Check sheet for the modelled part. Datum: model origin and axes. Units: mm. Face numbers are marked on the shaded views. A direction names the side the tool comes from. Give positions to 0.01 mm unless a question says otherwise; leave off trailing zeros. Order: outer loops, then holes, each group sorted by start corner. A loop starts at its lowest first (then second) coordinate and runs counter-clockwise, first axis right, second up. Notation, with made-up numbers: (-7.5, -0.75) -> (7.5, -0.75) arc R5 ccw to (7.5, 6.25) -> close; hole circle Ø9 at (44, 86.5). An arc over 180 degrees is marked (long way). Answer in a Markdown table with one row per item. Add a question column.
(1) Cross-section at B-B (y = 37). Record the cut outline in (x, z), then the cut area to 3 significant figures.
(2) Release check for a two-part mould opening along X. For the marked faces 3, 4, 5 and 6 record: released by +X, released by -X, zero draft, split by the parting line, or undercut.
(3) Cross-section at D-D (z = 7). Record the cut outline in (x, y), then the cut area to 3 significant figures.
(4) Cross-section at C-C (x = 0). Record the cut outline in (y, z).
(5) Cross-section at A-A (x = 7). Record the cut outline in (y, z).
(6) Set-up check for the marked faces 1 and 2: record each of +Z, -Z, +X, -X, +Y, -Y from which the full face is reachable in a straight line by a thin tool's end or side.
(7) Go/stop test with flat-tipped pins: pin 1 (3 mm diameter, centred on x = 0, z = -7, fed in from +Y); pin 2 (3 mm diameter, centred on y = 30, z = 7, fed in from +X). Record where each tip stops, or that it passes through.
(8) Thickness scan on L1, parallel to X at y = 22, z = -11; L2, parallel to Z at x = 7, y = 0.65; L3, parallel to Y at x = 13.5, z = 8.25. Record the ranges inside material, lowest first. Write a range as [from, to].
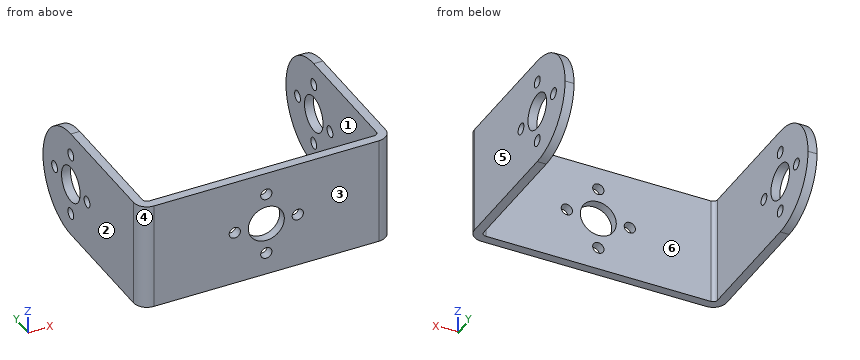
```python
from build123d import *

# Parameters (mm, degrees)
T_LE_DE_BASE_PLI_E1_DEPTH       = 12
ENL_V_START                     = -56
ENL_V_MAT_EXTRU_1_DEPTH         = 56
DIAM_TRE_DU_PER_AGE_8_0_8_1_D   = 8
DIAM_TRE_DU_PER_AGE_2_5_2_5_1_D = 2.5
DIAM_TRE_DU_PER_AGE_8_0_8_2_D   = 8
DIAM_TRE_DU_PER_AGE_2_5_2_5_2_D = 2.5


# Read off the part's stored shape, not the designer's step: Enlèv. mat.-Extru.1
# Sheet-metal steps are written as plain solids
with BuildPart() as part:
    # Esquisse1 → Tôle de base pliée1 (new, symmetric)
    with BuildSketch(Plane.XY):
        with BuildLine():
            Line((-28, 42), (-28, 3))
            ThreePointArc((-28, 3), (-27.121320344, 0.878679656), (-25, 0))
            Line((-25, 0), (25, 0))
            ThreePointArc((25, 0), (27.121320344, 0.878679656), (28, 3))
            Line((28, 3), (28, 42))
            Line((28, 42), (26, 42))
            Line((26, 42), (26, 3))
            ThreePointArc((26, 3), (25.707106781, 2.292893219), (25, 2))
            Line((25, 2), (-25, 2))
            ThreePointArc((-25, 2), (-25.707106781, 2.292893219), (-26, 3))
            Line((-26, 3), (-26, 42))
            Line((-26, 42), (-28, 42))
        make_face()
    extrude(amount=T_LE_DE_BASE_PLI_E1_DEPTH, both=True)

    # Enlèv. mat.-Extru.1 outline → Enlèv. mat.-Extru.1 (cut)
    with BuildSketch(Plane(origin=(28, 0, 0), x_dir=(0, 0, -1), z_dir=(1, 0, 0)).offset(ENL_V_START)):
        with BuildLine():
            ThreePointArc((-12, 30), (-8.485281374, 38.485281374), (0, 42))
            Line((0, 42), (-12, 42))
            Line((-12, 42), (-12, 30))
        make_face()
        with BuildLine():
            ThreePointArc((0, 42), (8.485281374, 38.485281374), (12, 30))
            Line((12, 30), (12, 42))
            Line((12, 42), (0, 42))
        make_face()
    extrude(amount=ENL_V_MAT_EXTRU_1_DEPTH, mode=Mode.SUBTRACT)

    # Diamètre du perçage Ø8.0 (8)1 (through all)
    with Locations(Plane(origin=(28, 0, 0), x_dir=(0, 0, -1), z_dir=(1, 0, 0))):
        with Locations((0, 30)):
            Hole(DIAM_TRE_DU_PER_AGE_8_0_8_1_D / 2)

    # Diamètre du perçage Ø2.5 (2.5)1 (through all)
    with Locations(Plane(origin=(28, 0, 0), x_dir=(0, 0, -1), z_dir=(1, 0, 0))):
        with Locations((0, 37), (7, 30), (0, 23), (-7, 30)):
            Hole(DIAM_TRE_DU_PER_AGE_2_5_2_5_1_D / 2)

    # Diamètre du perçage Ø8.0 (8)2 (through all)
    with Locations(Plane(origin=(0, 2, 0), x_dir=(1, 0, 0), z_dir=(0, 1, 0))):
        with Locations((0, 0)):
            Hole(DIAM_TRE_DU_PER_AGE_8_0_8_2_D / 2)

    # Diamètre du perçage Ø2.5 (2.5)2 (through all)
    with Locations(Plane(origin=(0, 2, 0), x_dir=(1, 0, 0), z_dir=(0, 1, 0))):
        with Locations((0, 7), (7, 0), (0, -7), (-7, 0)):
            Hole(DIAM_TRE_DU_PER_AGE_2_5_2_5_2_D / 2)


solid = part.part
```
Answer below:
| question | item | result |
|---|---|---|
| 1 | outline | (-28, -9.75) -> (-26, -9.75) -> (-26, -1.25) -> (-28, -1.25) -> close; (-28, 1.25) -> (-26, 1.25) -> (-26, 9.75) -> (-28, 9.75) -> close; (26, -9.75) -> (28, -9.75) -> (28, -1.25) -> (26, -1.25) -> close; (26, 1.25) -> (28, 1.25) -> (28, 9.75) -> (26, 9.75) -> close |
| 1 | area | 68.0 mm² |
| 2 | face 3 | zero draft |
| 2 | face 4 | released by -X |
| 2 | face 5 | released by +X |
| 2 | face 6 | undercut |
| 3 | outline | (-28, 3) arc R3 ccw to (-25, 0) -> (-1.25, 0) -> (-1.25, 2) -> (-25, 2) arc R1 cw to (-26, 3) -> (-26, 28.75) -> (-28, 28.75) -> close; (-28, 31.25) -> (-26, 31.25) -> (-26, 39.75) -> (-28, 39.75) -> close; (1.25, 0) -> (25, 0) arc R3 ccw to (28, 3) -> (28, 28.75) -> (26, 28.75) -> (26, 3) arc R1 cw to (25, 2) -> (1.25, 2) -> close; (26, 31.25) -> (28, 31.25) -> (28, 39.75) -> (26, 39.75) -> close |
| 3 | area | 245 mm² |
| 4 | outline | (0, -12) -> (2, -12) -> (2, -8.25) -> (0, -8.25) -> close; (0, -5.75) -> (2, -5.75) -> (2, -4) -> (0, -4) -> close; (0, 4) -> (2, 4) -> (2, 5.75) -> (0, 5.75) -> close; (0, 8.25) -> (2, 8.25) -> (2, 12) -> (0, 12) -> close |
| 5 | outline | (0, -12) -> (2, -12) -> (2, -1.25) -> (0, -1.25) -> close; (0, 1.25) -> (2, 1.25) -> (2, 12) -> (0, 12) -> close |
| 6 | face 1 | +Z, -Z, +Y |
| 6 | face 2 | +Z, -Z, -X, +Y, -Y |
| 7 | pin 1 | stops at y = 2 |
| 7 | pin 2 | stops at x = 28 |
| 8 | L1 | x = [-28, -26], [26, 28] |
| 8 | L2 | z = [-12, -1.25], [1.25, 12] |
| 8 | L3 | y = [0, 2] |
